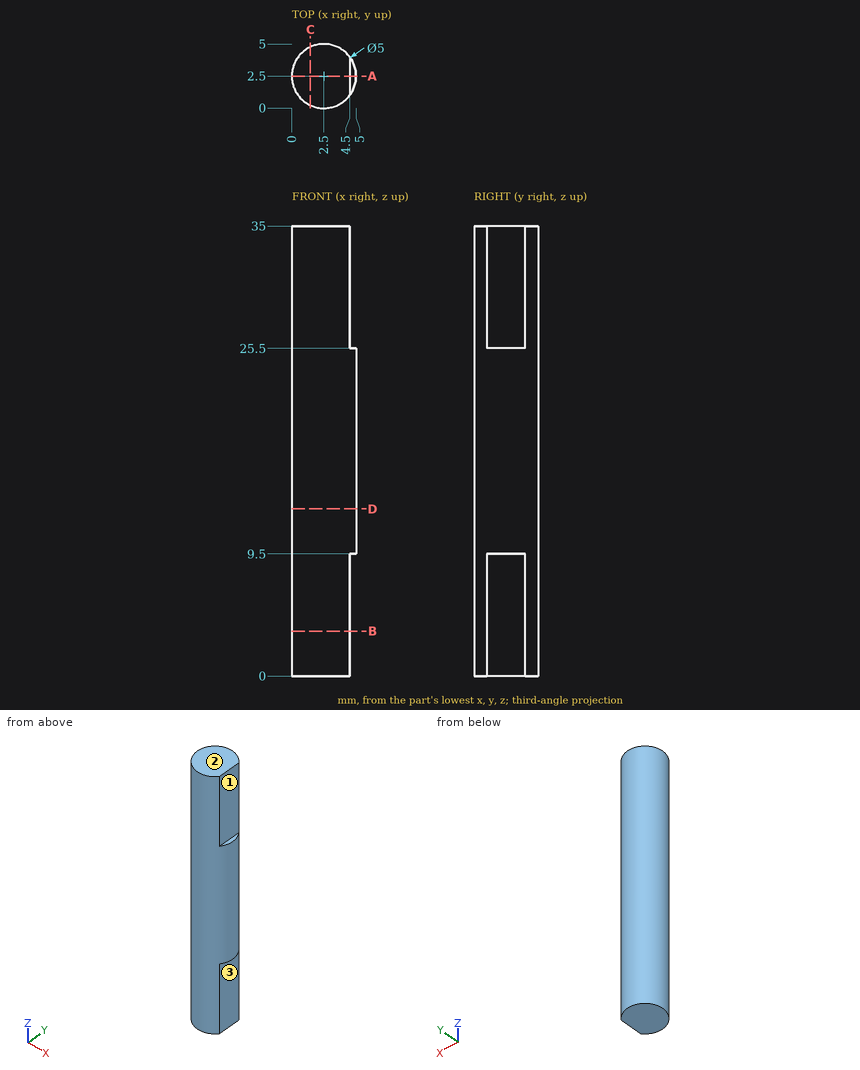
Verification items for this drawing (mm, ordinates from the low corner). A direction names the side the tool comes from. Give positions to 0.01 mm unless a question says otherwise; leave off trailing zeros. Loops run counter-clockwise (first coordinate to the right, second up) from the corner with the lowest first, then second, coordinate; pieces in that order, holes last.
1. Cross-section at A-A on y = 2.5. Record the cut outline in (x, z).
Derived:
outline: (0, 0) - (4.5, 0) - (4.5, 9.5) - (5, 9.5) - (5, 25.5) - (4.5, 25.5) - (4.5, 35) - (0, 35) - close
2. Cross-section at B-B on z = 3.5. Record the cut outline in (x, y), and give its area (3 significant figures).
Derived:
outline: (4.5, 1) - (4.5, 4) arc R2.5 ccw (long way) to start
area: 18.6 mm2
3. Cross-section at C-C on x = 1.45. Record the cut outline in (y, z), and give its area (3 significant figures).
Derived:
outline: (0.23, 0) - (4.77, 0) - (4.77, 35) - (0.23, 35) - close
area: 159 mm2
4. Cross-section at D-D on z = 13. Record the cut outline in (x, y), and give its area (3 significant figures).
Derived:
outline: circle Ø5 at (2.5, 2.5)
area: 19.6 mm2
5. Material ranges on probe 1 along Y at (x, z) = (2.6, 18); probe 2 along Z at (x, y) = (4.6, 1.7); probe 3 along Y at (x, z) = (0.5, 8), recorded low to high.
Derived:
probe 1: y = 0 to 5
probe 2: z = 9.5 to 25.5
probe 3: y = 1 to 4
6. Tool access check on the marked faces 1, 2 and 3. Record the directions out of +Z, -Z, +X, -X, +Y, -Y that give a thin tool (end or side, any length) a straight path to the whole face; none if there is none.
Derived:
face 1: +Z, +X, +Y, -Y
face 2: +Z, +X, -X, +Y, -Y
face 3: -Z, +X, +Y, -Y
